For this review, take the finished solid that the model builds, in its own axes (mm). Face numbers are marked on the shaded views. A direction names the side the tool comes from. Round coordinates to 2 decimals unless told otherwise and drop trailing zeros. Write each loop counter-clockwise with the first axis right and the second up, starting at its lowest first coordinate (ties: lowest second). Pieces come first, ordered by that corner, then holes. Notation, with made-up numbers: (-40, -34.5) - (-2, -34.5) arc R36 ccw to (-2, 2.5) - close; hole circle Ø7 at (22, -23). An arc over 180 degrees is marked (long way). One line per item, written item: value. Start each with the question number.
Q1. Tool access review of the marked faces 1, 2, 3 and 4: name each direction out of +Z, -Z, +X, -X, +Y, -Y from which nothing blocks a thin tool from reaching the whole face with its end or side.
Q2. Clearance check with flat-ended pins moving along their axes: pin 1 Ø4 at (y, z) = (7, -1.5) entering from -X (3 decimals); pin 2 Ø4 at (x, y) = (14.5, 15) entering from -Z; pin 3 Ø5 at (y, z) = (8.5, 15) entering from +X. State where each tip first meets the part, or that it passes through.
Q3. Add section A-A on z = 0. Write out the cut boundary in (x, y) (3 decimals).
Q4. For probe 1 along X at (y, z) = (0.35, 0) (3 decimals); probe 2 along Z at (x, y) = (-17.49, 0.65) (3 decimals); probe 3 along Y at (x, z) = (6, 14.5), list the stretches that pass through material, from the lowest coordinate up.
Q5. Add section D-D on x = 0. Write out the cut boundary in (y, z) (3 decimals).
Q6. Add section B-B on x = 16.5. Write out the cut boundary in (y, z) (3 decimals).
Q7. Add section C-C on y = -6.75. Write out the cut boundary in (x, z).
```python
from build123d import *
from build123d.topology import SkipClean

# Parameters (mm, degrees)
EXTRUDE_1_DEPTH = 19.05
SKETCH_2_R      = 2.0828
EXTRUDE_2_DEPTH = 0.889
SKETCH_3_R      = 4.635
EXTRUDE_3_DEPTH = 1.524
SKETCH_4_R      = 2.4892
EXTRUDE_4_DEPTH = 0.8001
EXTRUDE_5_DEPTH = 6.1976


with BuildPart() as part:
    # 스케치1 → 보스-돌출1 (new body)
    with BuildSketch(Plane(origin=(0, 0, 0), x_dir=(1, 0, 0), z_dir=(0, 1, 0))):
        with BuildLine():
            Line((-7.14375, -16.545), (7.14375, -16.545))
            Line((7.14375, -16.545), (7.14375, -12.092512598))
            ThreePointArc((7.14375, -12.092512598), (0, 14.045), (-7.14375, -12.092512598))
            Line((-7.14375, -12.092512598), (-7.14375, -16.545))
        make_face()
    extrude(amount=EXTRUDE_1_DEPTH)

    # 스케치2 → 보스-돌출2 (add)
    # profile 1 of 2: a face of its own
    with BuildSketch(Plane.XZ):
        with BuildLine():
            Line((-17.49, 3.475), (-13.608320984, 3.475))
            ThreePointArc((-13.608320984, 3.475), (-14.045, 0), (-13.608320984, -3.475))
            Line((-13.608320984, -3.475), (-17.49, -3.475))
            ThreePointArc((-17.49, -3.475), (-20.965, 0), (-17.49, 3.475))
        make_face()
        with Locations(Location((-17.49, 0, 0), (0, 0, 90))):
            Circle(SKETCH_2_R, mode=Mode.SUBTRACT)
    # profile 2 of 2: a face of its own
    with BuildSketch(Plane.XZ):
        with BuildLine():
            Line((17.49, 3.475), (13.608320984, 3.475))
            ThreePointArc((13.608320984, 3.475), (14.045, 0), (13.608320984, -3.475))
            Line((13.608320984, -3.475), (17.49, -3.475))
            ThreePointArc((17.49, -3.475), (20.965, 0), (17.49, 3.475))
        make_face()
        with Locations(Location((17.49, 0, 0), (0, 0, 270))):
            Circle(SKETCH_2_R, mode=Mode.SUBTRACT)
    extrude(amount=-EXTRUDE_2_DEPTH)

    # 스케치3 → 보스-돌출3 (add)
    with BuildSketch(Plane.XZ):
        with Locations(Location((0, -8.03, 0), (0, 0, 90))):
            Circle(SKETCH_3_R)
    extrude(amount=EXTRUDE_3_DEPTH)

    # 스케치4 → 보스-돌출4 (add)
    with BuildSketch(Plane.XZ.offset(1.524)):
        with Locations(Location((0, -8.03, 0), (0, 0, 270))):
            Circle(SKETCH_4_R)
    extrude(amount=EXTRUDE_4_DEPTH)

    # 스케치5 → 보스-돌출5 (add)
    with SkipClean():  # the faces are left unmerged after this step: merging them gives an invalid solid
        with BuildSketch(Plane.XZ.offset(2.3241)):
            with BuildLine():
                Line((2.001761334, -9.50955), (-2.001761334, -9.50955))
                ThreePointArc((-2.001761334, -9.50955), (-2.4892, -8.03), (-2.001761334, -6.55045))
                Line((-2.001761334, -6.55045), (2.001761334, -6.55045))
                ThreePointArc((2.001761334, -6.55045), (2.4892, -8.03), (2.001761334, -9.50955))
            make_face()
        extrude(amount=EXTRUDE_5_DEPTH)


solid = part.part
```
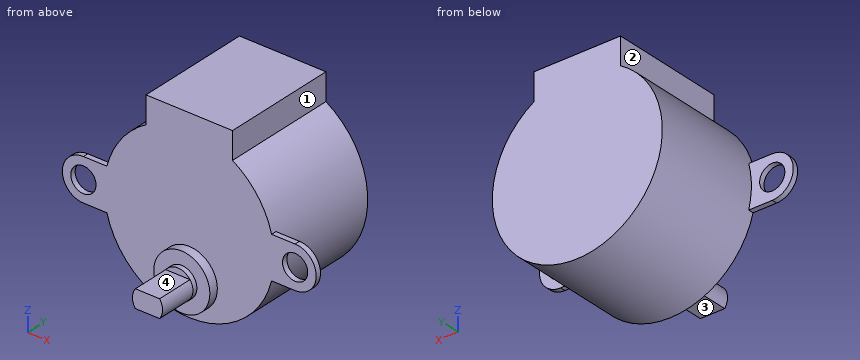
Result set:
1. face 1: +Z, +X, +Y, -Y
1. face 2: +Z, -X, +Y, -Y
1. face 3: -Z, +X, -X, -Y
1. face 4: +Z, +X, -X, -Y
2. pin 1: stops at x = -14.045
2. pin 2: stops at z = -6.4
2. pin 3: stops at x = 7.14
3. outline: (-20.965, 0) - (-19.573, 0) - (-19.573, 0.889) - (-20.965, 0.889) - close; (-15.407, 0) - (15.407, 0) - (15.407, 0.889) - (14.045, 0.889) - (14.045, 19.05) - (-14.045, 19.05) - (-14.045, 0.889) - (-15.407, 0.889) - close; (19.573, 0) - (20.965, 0) - (20.965, 0.889) - (19.573, 0.889) - close
4. probe 1: x = -20.965 to -19.573, -15.407 to 15.407, 19.573 to 20.965
4. probe 2: z = -3.475 to -2.083, 2.083 to 3.475
4. probe 3: y = 0 to 19.05
5. outline: (-8.522, -9.51) - (-2.324, -9.51) - (-2.324, -10.519) - (-1.524, -10.519) - (-1.524, -12.665) - (0, -12.665) - (0, -14.045) - (19.05, -14.045) - (19.05, 16.545) - (0, 16.545) - (0, -3.395) - (-1.524, -3.395) - (-1.524, -5.541) - (-2.324, -5.541) - (-2.324, -6.55) - (-8.522, -6.55) - close
6. outline: (0, -3.475) - (0.889, -3.475) - (0.889, -1.832) - (0, -1.832) - close; (0, 1.832) - (0.889, 1.832) - (0.889, 3.475) - (0, 3.475) - close
7. outline: (-2, -9.51) - (2, -9.51) arc R2.49 ccw to (2, -6.55) - (-2, -6.55) arc R2.49 ccw to start
